The model under review builds one solid part; all positions refer to its coordinate system, in mm. Round coordinates to 2 decimals unless told otherwise and drop trailing zeros. Write each loop counter-clockwise with the first axis right and the second up, starting at its lowest first coordinate (ties: lowest second). Pieces come first, ordered by that corner, then holes. Notation, with made-up numbers: M 58.5,79 L 114.5,79 A33 ccw 114.5,112 Z; hole C 38,72.25 d10. An arc over 180 degrees is marked long. One line per item, written item: value. Start each with the question number.
1) Wall thickness on probe 1 along Z at (x, y) = (-143.5, 3); probe 2 along Z at (x, y) = (-158.5, 0.2); probe 3 along X at (y, z) = (2.7, -35): over which ranges is each line inside the solid? List them lowest first.
2) Take a section at A-A, the plane z = -41. Write out the cut boundary in (x, y).
3) For P1, Ø1.5, axis at y = 2, z = -99, coming from the -X side; P2, Ø1.2, axis at y = 1, z = -37, coming from the -X side; P3, Ø1.5, axis at y = 2, z = -25, coming from the -X side, all flat-tipped, find the tip position at first contact; note any pin that passes through.
4) Take a section at D-D, the plane z = 21. Write out the cut boundary in (x, y), and give its area (3 significant figures).
5) Take a section at C-C, the plane y = 2.2. State how many separate pieces and enclosed holes the cut face has, and give its area (3 significant figures).
6) Take a section at B-B, the plane z = -65. Write out the cut boundary in (x, y).
from build123d import *

# Parameters (mm, degrees)
SKETCH1_R           = 1.6
SKETCH1_W           = 50
SKETCH1_H           = 50
SKETCH1_W_2         = 15
SKETCH1_H_2         = 3
SKETCH1_W_3         = 3
SKETCH1_H_3         = 15
BOSS_EXTRUDE1_DEPTH = 4


with BuildPart() as part:
    # Sketch1 → Boss-Extrude1 (new body)
    with BuildSketch(Plane(origin=(37.559096252, 0, 0), x_dir=(1, 0, 0), z_dir=(0, 1, 0))):
        with BuildLine():
            Line((48.217114977, 152.653937947), (48.217114977, -47.346062053))
            Line((48.217114977, -47.346062053), (-211.782885023, -47.346062053))
            ThreePointArc((-211.782885023, -47.346062053), (-240.105339993, -0.869375518), (-249.979486148, 52.653937947))
            ThreePointArc((-249.979486148, 52.653937947), (-240.105339993, 106.177251413), (-211.782885023, 152.653937947))
            Line((-211.782885023, 152.653937947), (48.217114977, 152.653937947))
        make_face()
        with Locations(Location((-198.353137603, 19.653937947, 0), (0, 0, 270))):
            Circle(SKETCH1_R, mode=Mode.SUBTRACT)
        with Locations(Location((-151.605834694, 19.653937947, 0), (0, 0, 90))):
            Circle(SKETCH1_R, mode=Mode.SUBTRACT)
        with Locations(Location((-198.353137603, 85.653937947, 0), (0, 0, 90))):
            Circle(SKETCH1_R, mode=Mode.SUBTRACT)
        with Locations(Location((-151.605834694, 85.653937947, 0), (0, 0, 270))):
            Circle(SKETCH1_R, mode=Mode.SUBTRACT)
        with Locations((-174.979486148, 52.653937947)):
            Rectangle(SKETCH1_W, SKETCH1_H, mode=Mode.SUBTRACT)
        with Locations((-187.479486148, 80.653937947)):
            Rectangle(SKETCH1_W_2, SKETCH1_H_2, mode=Mode.SUBTRACT)
        with Locations((-187.479486148, 24.653937947)):
            Rectangle(SKETCH1_W_2, SKETCH1_H_2, mode=Mode.SUBTRACT)
        with Locations((-162.479486148, 24.653937947)):
            Rectangle(SKETCH1_W_2, SKETCH1_H_2, mode=Mode.SUBTRACT)
        with Locations((-162.479486148, 80.653937947)):
            Rectangle(SKETCH1_W_2, SKETCH1_H_2, mode=Mode.SUBTRACT)
        with Locations((-146.979486148, 40.153937947)):
            Rectangle(SKETCH1_W_3, SKETCH1_H_3, mode=Mode.SUBTRACT)
        with Locations((-146.979486148, 65.153937947)):
            Rectangle(SKETCH1_W_3, SKETCH1_H_3, mode=Mode.SUBTRACT)
        with Locations((-202.979486148, 40.153937947)):
            Rectangle(SKETCH1_W_3, SKETCH1_H_3, mode=Mode.SUBTRACT)
        with Locations((-202.979486148, 65.153937947)):
            Rectangle(SKETCH1_W_3, SKETCH1_H_3, mode=Mode.SUBTRACT)
    extrude(amount=BOSS_EXTRUDE1_DEPTH)


solid = part.part
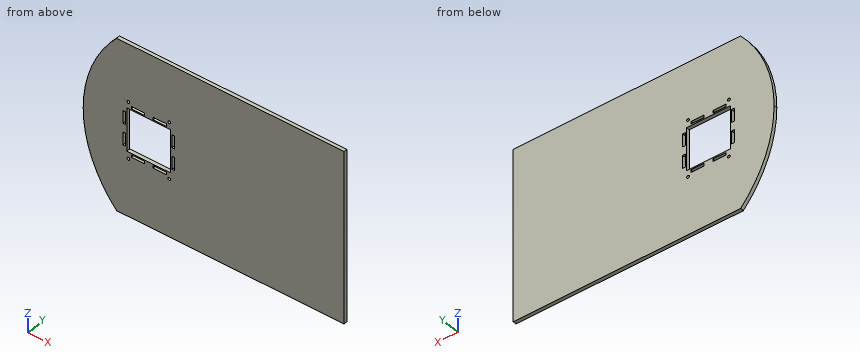
Checked values:
1. probe 1: z = -152.65 to -82.15, -79.15 to -77.65, -27.65 to -26.15, -23.15 to 47.35
1. probe 2: z = -152.65 to -77.65, -27.65 to 47.35
1. probe 3: x = -211.38 to -166.92, -163.92 to -162.42, -112.42 to -110.92, -107.92 to 85.78
2. outline: M -211.97,0 L -166.92,0 L -166.92,4 L -211.97,4 Z; M -163.92,0 L -162.42,0 L -162.42,4 L -163.92,4 Z; M -112.42,0 L -110.92,0 L -110.92,4 L -112.42,4 Z; M -107.92,0 L 85.78,0 L 85.78,4 L -107.92,4 Z
3. P1: stops at x = -205.32
3. P2: stops at x = -211.66
3. P3: stops at x = -209.99
4. outline: M -193.09,0 L 85.78,0 L 85.78,4 L -193.09,4 Z
4. area: 1,120 mm2
5. separate pieces: 1
5. enclosed holes: 13
5. area: 54,300 mm2
6. outline: M -211.91,0 L -166.92,0 L -166.92,4 L -211.91,4 Z; M -163.92,0 L -162.42,0 L -162.42,4 L -163.92,4 Z; M -112.42,0 L -110.92,0 L -110.92,4 L -112.42,4 Z; M -107.92,0 L 85.78,0 L 85.78,4 L -107.92,4 Z
